Check sheet for the modelled part. Datum: model origin and axes. Units: mm. Round coordinates to 2 decimals unless told otherwise and drop trailing zeros.
from build123d import *

# Parameters (mm, degrees)
SKETCH1_W           = 508
SKETCH1_H           = 304.8
SKETCH1_W_2         = 50.8
SKETCH1_H_2         = 6.35
SKETCH1_W_3         = 3.175
SKETCH1_H_3         = 12.7
BOSS_EXTRUDE1_DEPTH = 3.175
SKETCH2_R           = 1.5
SKETCH2_R_2         = 1.499997
CUT_EXTRUDE1_DEPTH  = 3.175


with BuildPart() as part:
    # Sketch1 → Boss-Extrude1 (new body)
    with BuildSketch(Plane.XY):
        with Locations((254, 152.4)):
            Rectangle(SKETCH1_W, SKETCH1_H)
        with Locations((50.8, -3.175)):
            Rectangle(SKETCH1_W_2, SKETCH1_H_2)
        with Locations((152.4, -3.175)):
            Rectangle(SKETCH1_W_2, SKETCH1_H_2)
        with Locations((254, -3.175)):
            Rectangle(SKETCH1_W_2, SKETCH1_H_2)
        with Locations((355.6, -3.175)):
            Rectangle(SKETCH1_W_2, SKETCH1_H_2)
        with Locations((457.2, -3.175)):
            Rectangle(SKETCH1_W_2, SKETCH1_H_2)
        with Locations((-1.5875, 19.05)):
            Rectangle(SKETCH1_W_3, SKETCH1_H_3)
        with Locations((-1.5875, 44.45)):
            Rectangle(SKETCH1_W_3, SKETCH1_H_3)
        with Locations((-1.5875, 69.85)):
            Rectangle(SKETCH1_W_3, SKETCH1_H_3)
        with Locations((-1.5875, 95.25)):
            Rectangle(SKETCH1_W_3, SKETCH1_H_3)
        with Locations((-1.5875, 120.65)):
            Rectangle(SKETCH1_W_3, SKETCH1_H_3)
        with Locations((-1.5875, 146.05)):
            Rectangle(SKETCH1_W_3, SKETCH1_H_3)
        with Locations((-1.5875, 171.45)):
            Rectangle(SKETCH1_W_3, SKETCH1_H_3)
        with Locations((-1.5875, 196.85)):
            Rectangle(SKETCH1_W_3, SKETCH1_H_3)
        with Locations((-1.5875, 222.25)):
            Rectangle(SKETCH1_W_3, SKETCH1_H_3)
        with Locations((-1.5875, 247.65)):
            Rectangle(SKETCH1_W_3, SKETCH1_H_3)
        with Locations((-1.5875, 273.05)):
            Rectangle(SKETCH1_W_3, SKETCH1_H_3)
        with Locations((-1.5875, 298.45)):
            Rectangle(SKETCH1_W_3, SKETCH1_H_3)
        with Locations((509.5875, 19.05)):
            Rectangle(SKETCH1_W_3, SKETCH1_H_3)
        with Locations((509.5875, 44.45)):
            Rectangle(SKETCH1_W_3, SKETCH1_H_3)
        with Locations((509.5875, 69.85)):
            Rectangle(SKETCH1_W_3, SKETCH1_H_3)
        with Locations((509.5875, 95.25)):
            Rectangle(SKETCH1_W_3, SKETCH1_H_3)
        with Locations((509.5875, 146.05)):
            Rectangle(SKETCH1_W_3, SKETCH1_H_3)
        with Locations((509.5875, 120.65)):
            Rectangle(SKETCH1_W_3, SKETCH1_H_3)
        with Locations((509.5875, 171.45)):
            Rectangle(SKETCH1_W_3, SKETCH1_H_3)
        with Locations((509.5875, 196.85)):
            Rectangle(SKETCH1_W_3, SKETCH1_H_3)
        with Locations((509.5875, 222.25)):
            Rectangle(SKETCH1_W_3, SKETCH1_H_3)
        with Locations((509.5875, 247.65)):
            Rectangle(SKETCH1_W_3, SKETCH1_H_3)
        with Locations((509.5875, 273.05)):
            Rectangle(SKETCH1_W_3, SKETCH1_H_3)
        with Locations((509.5875, 298.45)):
            Rectangle(SKETCH1_W_3, SKETCH1_H_3)
    extrude(amount=BOSS_EXTRUDE1_DEPTH)

    # Sketch2 → Cut-Extrude1 (cut)
    with BuildSketch(Plane.XY.offset(3.175)):
        with Locations((15.875, 289.8)):
            Circle(SKETCH2_R)
        with Locations((15.875, 274.05)):
            Circle(SKETCH2_R_2)
        with Locations((492.125, 289.8)):
            Circle(SKETCH2_R)
        with Locations((492.125, 274.05)):
            Circle(SKETCH2_R_2)
    extrude(amount=-CUT_EXTRUDE1_DEPTH, mode=Mode.SUBTRACT)


solid = part.part
1. Scan lines: line 1 along X through (y, z) = (274.05, 2.1) (3 decimals); line 2 along X through (y, z) = (289.8, 2.05) (3 decimals); line 3 along Y through (x, z) = (181.5, 2.9). Record each from-to range of solid material in increasing order.
2. Go/stop test with flat-tipped pins: pin 1 (1.6 mm diameter, centred on x = -1.5, z = 2, fed in from -Y); pin 2 (1 mm diameter, centred on y = 57.5, z = 1.5, fed in from -X); pin 3 (1 mm diameter, centred on y = 157, z = 1, fed in from +X); pin 4 (4 mm diameter, centred on x = 227, y = 261.5, fed in from -Z). Record where each tip stops, or that it passes through.
3. Sectioned sample at A-A, the plane z = 1. Give the number of separate pieces and of enclosed holes in the cut face, plus the area to 3 significant figures.
Computed values:
1. line 1: x = -3.175 to 14.375, 17.375 to 490.625, 493.625 to 511.175
1. line 2: x = 0 to 14.375, 17.375 to 490.625, 493.625 to 508
1. line 3: y = 0 to 304.8
2. pin 1: stops at y = 12.7
2. pin 2: stops at x = 0
2. pin 3: stops at x = 508
2. pin 4: stops at z = 0
3. separate pieces: 1
3. enclosed holes: 4
3. area: 157,000 mm2
